Here's the drawing with two shaded views (mm, measured from the low corner). I have some questions. Give positions to 0.01 mm unless a question says otherwise; leave off trailing zeros. Write each loop counter-clockwise with the first axis right and the second up, starting at its lowest first coordinate (ties: lowest second). Pieces come first, ordered by that corner, then holes.
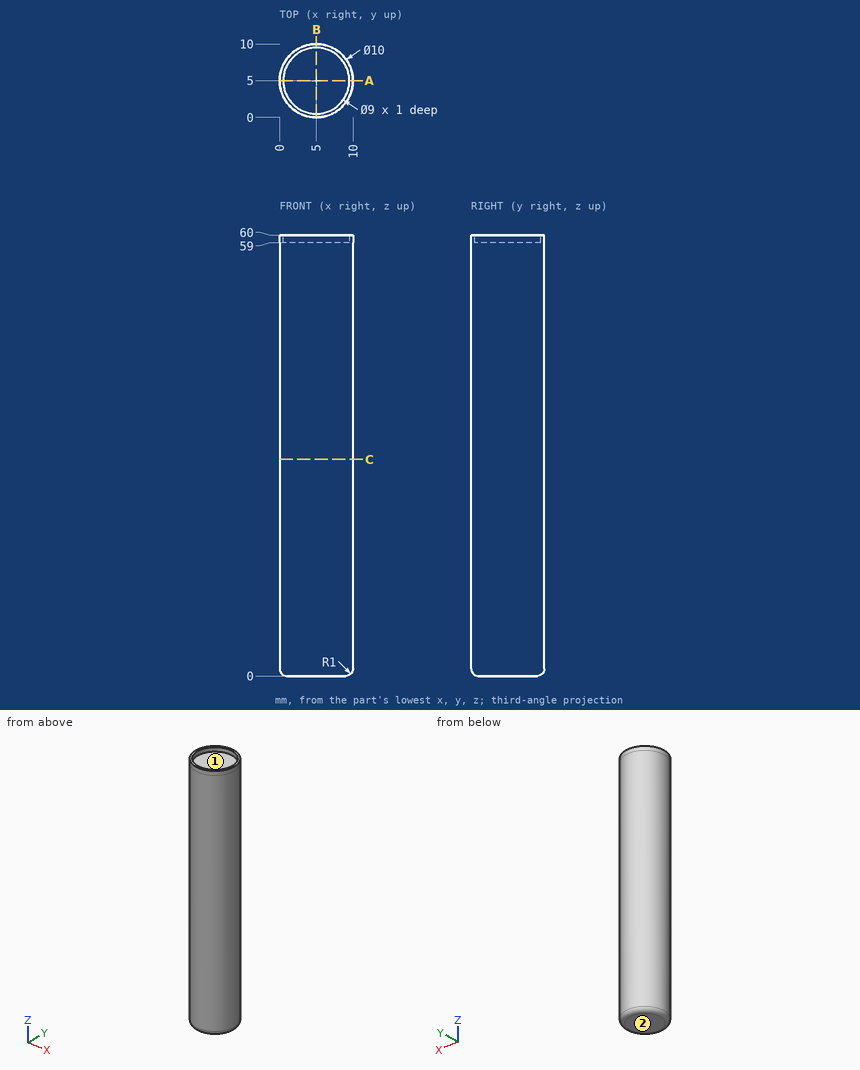
(1) Will these pins go through, and if not, where does the flat tip stop? P1, Ø2.5, axis at x = 7, y = 5.5, coming from the +Z side; P2, Ø1.5, axis at y = 7.5, z = 36.5, coming from the -X side; P3, Ø5, axis at x = 5.5, y = 7.5, coming from the -Z side; P4, Ø5, axis at y = 1.5, z = 41.5, coming from the -X side.
Returned:
P1: stops at z = 59
P2: stops at x = 0.32
P3: stops at z = 0
P4: stops at x = 0.1
(2) Imagine slicing it at A-A, the plane y = 5. Write out the boundary of the cut face in (x, z).
Returned:
outline: (0, 1) arc R1 ccw to (1, 0) - (9, 0) arc R1 ccw to (10, 1) - (10, 60) - (9.5, 60) - (9.5, 59) - (0.5, 59) - (0.5, 60) - (0, 60) - close
(3) If I drill on L1, parallel to Y at x = 5, z = 59.35; L2, parallel to Z at x = 7.5, y = 5.5; L3, parallel to Y at x = 2, z = 51, over which ranges is the centre line in solid material (lowest first)?
Returned:
L1: y = 0 to 0.5, 9.5 to 10
L2: z = 0 to 59
L3: y = 1 to 9
(4) Imagine slicing it at C-C, the plane z = 29.5. Write out the boundary of the cut face in (x, y).
Returned:
outline: circle Ø10 at (5, 5)
(5) If we mould it in two halves opening along Y, with no side actions, what happens to the marked faces 1 and 2? For each: +Y half, -Y half, draft (parallel to the pull), parting line (faces both ways), or undercut.
Returned:
face 1: undercut
face 2: draft
